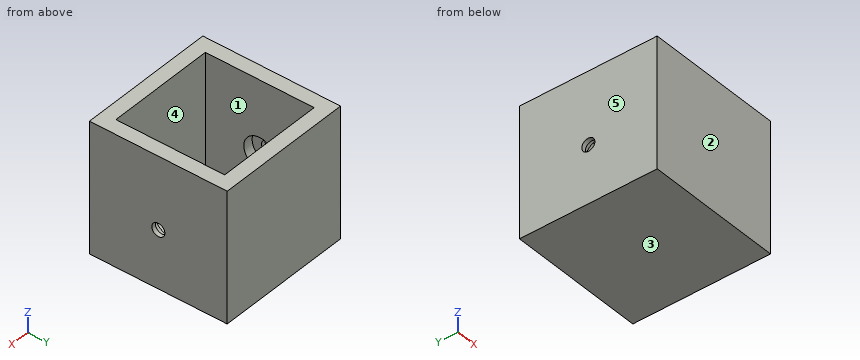
Autodesk Inventor part; units mm, degrees
ref_plane "YZ Plane" through (0, 0, 0) normal (1, 0, 0) x (0, 1, 0)
ref_plane "XZ Plane" through (0, 0, 0) normal (0, 1, 0) x (-1, 0, 0)
ref_plane "XY Plane" through (0, 0, 0) normal (0, 0, 1) x (1, 0, 0)
sketch "Sketch1" plane through (0, 0, 0) normal (0, 0, 1) x (1, 0, 0)
  line L0 (-37.5, -37.5) -> (37.5, -37.5)
  line L1 (37.5, -37.5) -> (37.5, 37.5)
  line L2 (37.5, 37.5) -> (-37.5, 37.5)
  line L3 (-37.5, 37.5) -> (-37.5, -37.5)
  line L4 (-37.5, -37.5) -> (37.5, 37.5) construction
  line L5 (37.5, -37.5) -> (-37.5, 37.5) construction
  line L6 (47.5, 47.5) -> (47.5, -47.5)
  line L7 (47.5, -47.5) -> (-47.5, -47.5)
  line L8 (-47.5, -47.5) -> (-47.5, 47.5)
  line L9 (-47.5, 47.5) -> (47.5, 47.5)
  point P0 (0, 0)
  dimension "d0" = 75
  dimension "d1" = 75
  dimension "d2" = 10
extrude "Extrusion1" add sketch "Sketch1" along normal blind 5 contours L3 L2 L1 L0 | L6 L7 L8 L9
extrude "Extrusion2" add sketch "Sketch1" along normal blind 90
sketch "Sketch5" plane through (-37.5, -37.5, 5) normal (1, 0, 0) x (0, 0, -1)
  circle A0 centre (-35, 37.5) radius 11
  line L0 (5, 85) -> (5, -10)
  circle A1 centre (-35, 37.5) radius 4.5
  point P0 (5, 37.5)
  point P1 (5, 37.5)
  dimension "d16" = 22
  dimension "d17" = 40
  dimension "d18" = 9
extrude "Extrusion5" cut sketch "Sketch5" against normal blind 7
extrude "Extrusion6" cut sketch "Sketch5" against normal up to surface (10 mm away) contours A1
mirror "Mirror2" about plane through (0, 0, 0) normal (1, 0, 0) of "Extrusion6", "Extrusion5"
properties part number "draaideel voor endeffector"
Geometry check sheet. Reference: the model listing, model coordinates, mm. Face numbers are marked on the shaded views. A direction names the side the tool comes from. Round coordinates to 2 decimals unless told otherwise and drop trailing zeros. Loops run counter-clockwise (first coordinate to the right, second up) from the corner with the lowest first, then second, coordinate; pieces in that order, holes last. Notation, with made-up numbers: (11, 12.5) - (19, 12.5) arc R28 cw to (19, 34.5) - close; hole circle Ø7 at (82, -5). An arc over 180 degrees is marked (long way). Write item = value, one per line. Start each with the question number.
1. Thickness scan on line 1 (X direction, y = 0.5, z = 73.5); line 2 (Y direction, x = 40, z = 40). Record the ranges inside material, lowest first.
2. Section check C-C on z = 40. Enter the section's corners in (x, y), then the cut area to 3 significant figures.
3. Depth check by flat-ended pin: pin 1 (12 mm diameter, centred on x = 20, y = -25.5, fed in from +Z). Enter the tip coordinate at first touch or a pass-through.
4. Section check B-B on z = 62. Enter the section's corners in (x, y), then the cut area to 3 significant figures.
5. Section check D-D on x = 1.5. Enter the section's corners in (y, z), then the cut area to 4 significant figures.
6. Mould release check, pull along X, two halves, no side actions. Record for the marked faces 3, 4 and 5: released by +X, released by -X, zero draft, split by the parting line, or undercut.
7. Set-up check for the marked faces 1 and 2: record each of +Z, -Z, +X, -X, +Y, -Y from which the full face is reachable in a straight line by a thin tool's end or side.
8. Section check A-A on y = 0. Enter the section's corners in (x, z).
Working result:
q1.line_1 = -47.5 to -37.5, 37.5 to 47.5
q1.line_2 = -47.5 to -11, 11 to 47.5
q2.outline = (-47.5, -47.5) - (47.5, -47.5) - (47.5, -4.5) - (44.5, -4.5) - (44.5, -11) - (37.5, -11) - (37.5, -37.5) - (-37.5, -37.5) - (-37.5, -11) - (-44.5, -11) - (-44.5, -4.5) - (-47.5, -4.5) - close; (-47.5, 4.5) - (-44.5, 4.5) - (-44.5, 11) - (-37.5, 11) - (-37.5, 37.5) - (37.5, 37.5) - (37.5, 11) - (44.5, 11) - (44.5, 4.5) - (47.5, 4.5) - (47.5, 47.5) - (-47.5, 47.5) - close
q2.area = 3,040 mm^2
q3.pin_1 = 5
q4.outline = (-47.5, -47.5) - (47.5, -47.5) - (47.5, 47.5) - (-47.5, 47.5) - close; hole (-37.5, -37.5) - (37.5, -37.5) - (37.5, 37.5) - (-37.5, 37.5) - close
q4.area = 3,400 mm^2
q5.outline = (-47.5, 0) - (47.5, 0) - (47.5, 90) - (37.5, 90) - (37.5, 5) - (-37.5, 5) - (-37.5, 90) - (-47.5, 90) - close
q5.area = 2,175 mm^2
q6.face_3 = zero draft
q6.face_4 = undercut
q6.face_5 = released by -X
q7.face_1 = +Z
q7.face_2 = +Z, -Z, +X, -X, -Y
q8.outline = (-47.5, 0) - (47.5, 0) - (47.5, 35.5) - (44.5, 35.5) - (44.5, 29) - (37.5, 29) - (37.5, 5) - (-37.5, 5) - (-37.5, 29) - (-44.5, 29) - (-44.5, 35.5) - (-47.5, 35.5) - close; (-47.5, 44.5) - (-44.5, 44.5) - (-44.5, 51) - (-37.5, 51) - (-37.5, 90) - (-47.5, 90) - close; (37.5, 51) - (44.5, 51) - (44.5, 44.5) - (47.5, 44.5) - (47.5, 90) - (37.5, 90) - close
